from build123d import *

# Parameters (mm, degrees)
F0_W      = 38.1
F0_H      = 60.325
F1_DEPTH  = 139.7
F2_W      = 34.925
F2_H      = 53.975
F3_DEPTH  = 762
F4_W      = 34.925
F4_H      = 31.75
F5_DEPTH  = 85.344
F6_R      = 9.525
F8_D      = 12.7
F8_DEPTH  = 127
F10_D     = 12.7
F10_DEPTH = 127


with BuildPart() as f1:
    # F0 (on Top) → F1 (new body)
    with BuildSketch(Plane.XY):
        with Locations((19.05, 30.1625)):
            Rectangle(F0_W, F0_H)
    extrude(amount=F1_DEPTH)

    # F2 (on face) → F3 (cut)
    with BuildSketch(Plane.XY.offset(139.7)):
        with Locations((20.6375, 30.1625)):
            Rectangle(F2_W, F2_H)
    extrude(amount=-F3_DEPTH, mode=Mode.SUBTRACT)

    # F4 (on face) → F5 (cut)
    with BuildSketch(Plane.XZ):
        with Locations((20.6375, 123.825)):
            Rectangle(F4_W, F4_H)
    extrude(amount=-F5_DEPTH, mode=Mode.SUBTRACT)

    # F6
    f6_edges = [f1.edges().sort_by_distance(p)[0] for p in [
        (3.175, 57.15, 53.975),
        (3.175, 3.175, 53.975),
        (0, 0, 69.85),
        (0, 60.325, 69.85),
    ]]
    fillet(f6_edges, radius=F6_R)

    # F8
    with Locations(Plane.XZ):
        with Locations((22.419682, 95.25), (22.419682, 12.7)):
            Hole(F8_D / 2, depth=F8_DEPTH)

    # F10
    with Locations(Plane.XZ):
        with Locations((22.419682, 69.85)):
            Hole(F10_D / 2, depth=F10_DEPTH)


solid = f1.part
Geometry: final body of the model. Coordinates: model frame, mm. A direction names the side the tool comes from. Round coordinates to 2 decimals unless told otherwise and drop trailing zeros. Loops run counter-clockwise (first coordinate to the right, second up) from the corner with the lowest first, then second, coordinate; pieces in that order, holes last. Notation, with made-up numbers: M -13.5,67.5 L -7.5,67.5 A21 ccw -7.5,103.5 Z; hole C 15,27 d4. An arc over 180 degrees is marked long. One line per question, with ' | ' between items.
(1) Cut plane A-A on z = 69.85. Return the cut outline in (x, y) (3 decimals), plus the area to 3 significant figures.
Check result:
outline: M 0,9.525 A9.525 ccw 9.525,0 L 16.07,0 L 16.07,3.175 L 12.7,3.175 A9.525 cw 3.175,12.7 L 3.175,47.625 A9.525 cw 12.7,57.15 L 16.07,57.15 L 16.07,60.325 L 9.525,60.325 A9.525 ccw 0,50.8 Z; M 28.77,0 L 38.1,0 L 38.1,3.175 L 28.77,3.175 Z; M 28.77,57.15 L 38.1,57.15 L 38.1,60.325 L 28.77,60.325 Z | area: 333 mm2
(2) Cut plane B-B on x = 33.5. Return the cut outline in (y, z) (3 decimals).
Check result:
outline: M 0,0 L 3.175,0 L 3.175,107.95 L 0,107.95 Z; M 57.15,0 L 60.325,0 L 60.325,107.95 L 57.15,107.95 Z
(3) Material intervals for line 1 along Y through (x, z) = (32.5, 58) (3 decimals); line 2 along X through (y, z) = (26.5, 19) (3 decimals); line 3 along Z through (x, y) = (5, 55), sorted ascending. Write a range as from..to.
Check result:
line 1: y = 0..3.175, 57.15..60.325 | line 2: x = 0..3.175 | line 3: z = 0..107.95
(4) Pull-direction query (Y, two-part tool) for faces 3 (the flat face through (25, 57.15, 55)), 4 (the flat face through (19, 58, 107.95)), 5 (the flat face through (24, 0, 53)); classes: +Y half, -Y half, draft (parallel to the pull), parting line (faces both ways), or undercut.
Check result:
face 3: undercut | face 4: draft | face 5: -Y half
(5) Contact query for flat-ended pins moving along their axis: P1, Ø10, axis at y = 46.5, z = 111.5, coming from the +X side; P2, Ø10, axis at x = 25, y = 5.5, coming from the +Z side; P3, Ø8, axis at y = 25, z = 16.5, coming from the +X side (3 decimals). Output: stop coordinate, or through.
Check result:
P1: stops at x = 3.48 | P2: stops at z = 107.95 | P3: stops at x = 3.175
(6) Cut plane D-D on z = 30.5. Return the cut outline in (x, y) (3 decimals), plus the area to 3 significant figures.
Check result:
outline: M 0,9.525 A9.525 ccw 9.525,0 L 38.1,0 L 38.1,3.175 L 12.7,3.175 A9.525 cw 3.175,12.7 L 3.175,47.625 A9.525 cw 12.7,57.15 L 38.1,57.15 L 38.1,60.325 L 9.525,60.325 A9.525 ccw 0,50.8 Z | area: 413 mm2
(7) Cut plane C-C on x = 19.5. Give the number of separate pieces and of enclosed holes in the cut face, plus the area to 3 significant figures.
Check result:
separate pieces: 8 | enclosed holes: 0 | area: 471 mm2
(8) Access query for faces 1 (the flat face through (25, 3.175, 55)), 2 (the cylindrical face through (27.1, 1.61, 16.99)). Directions: +Z, -Z, +X, -X, +Y, -Y. A direction counts if a zero-diameter tool reaches every point of the face in a straight line with its end or side. Return the directions, or none.
Check result:
face 1: +Z, -Z, +X | face 2: +Y, -Y
